Check sheet for the modelled part. Datum: model origin and axes. Units: mm. Face numbers are marked on the shaded views. A direction names the side the tool comes from. Round coordinates to 2 decimals unless told otherwise and drop trailing zeros. Order: outer loops, then holes, each group sorted by start corner. A loop starts at its lowest first (then second) coordinate and runs counter-clockwise, first axis right, second up.
(1) Thickness scan on probe 1 along Z at (x, y) = (-7, -21); probe 2 along Y at (x, z) = (-3, 71.5); probe 3 along X at (y, z) = (8, 66). Record the ranges inside material, lowest first.
(2) Sectioned sample at A-A, the plane y = 13. Enter the section's corners in (x, z), and give its area (3 significant figures).
(3) Depth check by flat-ended pin: pin 1 (2 mm diameter, centred on x = -12.5, y = 17.5, fed in from -Z); pin 2 (10 mm diameter, centred on x = 14.5, y = -7, fed in from +Z); pin 3 (19 mm diameter, centred on y = -18.5, z = 57, fed in from +X). Enter the tip coordinate at first touch or a pass-through.
(4) Sectioned sample at B-B, the plane x = -19.5. Enter the section's corners in (y, z), and give its area (3 significant figures).
(5) Sectioned sample at C-C, the plane z = 57.5. Enter the section's corners in (x, y).
(6) Tool access check on the marked faces 1 and 2. Record the directions out of +Z, -Z, +X, -X, +Y, -Y that give a thin tool (end or side, any length) a straight path to the whole face; none if there is none.
```python
from build123d import *

# Parameters (mm, degrees)
F0_W     = 101.6
F0_H     = 63.5
F1_DEPTH = 25.4
F3_DEPTH = 50.8
F5_DEPTH = 25.4


with BuildPart() as f1:
    # F0 (on Top) → F1 (new body)
    with BuildSketch(Plane.XY):
        with Locations((1.061673, 2.829394)):
            Rectangle(F0_W, F0_H)
    extrude(amount=F1_DEPTH)

    # F2 (on face) → F3 (join)
    with BuildSketch(Plane.XY.offset(25.4)):
        Polygon((-49.738327, 9.179394), (-49.738327, -28.920606), (-24.338327, -28.920606), (-24.338327, 9.179394), (1.061673, 9.179394), (1.061673, 34.579394), (-24.338327, 34.579394), (-49.738327, 34.579394), align=None)
    extrude(amount=F3_DEPTH)

    # F4 (on face) → F5 (join)
    with BuildSketch(Plane(origin=(0, 34.579394, 0), x_dir=(-1, 0, 0), z_dir=(0, 1, 0))):
        Polygon((-1.061673, 25.4), (-1.061673, 76.2), (-51.861673, 25.4), align=None)
    extrude(amount=-F5_DEPTH)


solid = f1.part
```
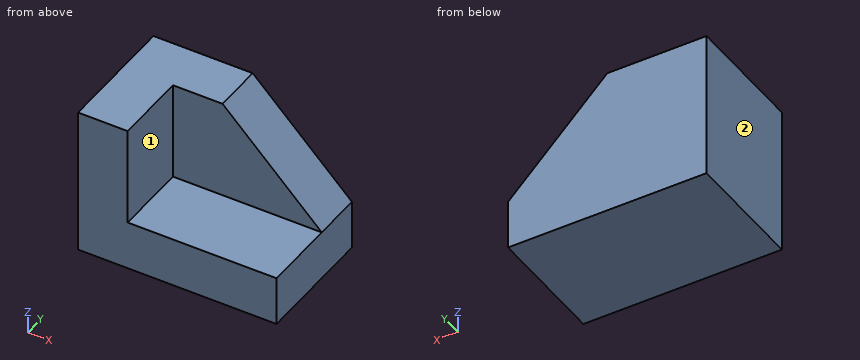
Derived:
1. probe 1: z = 0 to 25.4
1. probe 2: y = 9.18 to 34.58
1. probe 3: x = -49.74 to -24.34
2. outline: (-49.74, 0) - (51.86, 0) - (51.86, 25.4) - (1.06, 76.2) - (-49.74, 76.2) - close
2. area: 6,450 mm2
3. pin 1: stops at z = 0
3. pin 2: stops at z = 25.4
3. pin 3: stops at x = -24.34
4. outline: (-28.92, 0) - (34.58, 0) - (34.58, 76.2) - (9.18, 76.2) - (9.18, 25.4) - (-28.92, 25.4) - close
4. area: 2,900 mm2
5. outline: (-49.74, -28.92) - (-24.34, -28.92) - (-24.34, 9.18) - (19.76, 9.18) - (19.76, 34.58) - (-49.74, 34.58) - close
6. face 1: +Z, +X, -Y
6. face 2: +Z, -Z, -X, +Y, -Y
